The model under review builds one solid part; all positions refer to its coordinate system, in mm. A direction names the side the tool comes from. Give positions to 0.01 mm unless a question says otherwise; leave off trailing zeros. Order: outer loops, then holes, each group sorted by start corner. A loop starts at its lowest first (then second) coordinate and runs counter-clockwise, first axis right, second up.
```python
from build123d import *

# Parameters (mm, degrees)
F1_DEPTH    = 48
F2_DEPTH    = 10
F3_R        = 6.0205101074
F4_DEPTH    = 3
F5_T1_DEPTH = 30
F6_R        = 6


# Not quite as in the source:
# - a fillet or chamfer that OpenCascade refuses, or shapes differently, is made with other operations: its cross-section is extruded or revolved along the edge and cut away or added


with BuildPart() as f1:
    # F0 (on Top) → F1 (new body)
    with BuildSketch(Plane.XY):
        Polygon((20, 10), (0, 10), (-20, 10), (-20, 30), (-30, 30), (-30, 0), (0, 0), (30, 0), (30, 30), (20, 30), align=None)
    extrude(amount=F1_DEPTH)

    # F0 (on Top) → F2 (join)
    with BuildSketch(Plane.XY):
        Polygon((20, 10), (0, 10), (-20, 10), (-20, 30), (-30, 30), (-30, 0), (0, 0), (30, 0), (30, 30), (20, 30), align=None)
        Polygon((-30, 0), (-30, 30), (-45, 30), (-45, -18), (0, -18), (45, -18), (45, 30), (30, 30), (30, 0), (0, 0), align=None)
    extrude(amount=F2_DEPTH)

    # F3 (on Front) → F4 (join)
    with BuildSketch(Plane.XZ):
        with BuildLine():
            Line((14, 10), (14, 29))
            ThreePointArc((14, 29), (0, 43), (-14, 29))
            Line((-14, 29), (-14, 10))
            Line((-14, 10), (14, 10))
        make_face()
        with Locations((0, 29)):
            Circle(F3_R, mode=Mode.SUBTRACT)
    extrude(amount=F4_DEPTH)

    # F5: fillet of radius 25 on 2 edges, made by hand

    # F5_s2 → F5_t1 (join)
    with BuildSketch(Plane.XZ.offset(-30)):
        with BuildLine():
            ThreePointArc((30, 32.9128784748), (34.0834993366, 19.2198145372), (45, 10))
            Line((45, 10), (30, 10))
            Line((30, 10), (30, 32.9128784748))
        make_face()
        with BuildLine():
            ThreePointArc((-30, 32.9128784748), (-34.0834993366, 19.2198145372), (-45, 10))
            Line((-45, 10), (-30, 10))
            Line((-30, 10), (-30, 32.9128784748))
        make_face()
    extrude(amount=F5_T1_DEPTH)

    # F6
    f6_edges = [f1.edges().sort_by_distance(p)[0] for p in [
        (-45, -18, 5),
        (45, -18, 5),
    ]]
    fillet(f6_edges, radius=F6_R)


solid = f1.part
```
Item 1: Take a section at B-B (z = 3). Give the boundary of the cut face in (x, y), and give its area (3 significant figures).
Values found:
outline: (-45, -12) arc R6 ccw to (-39, -18) - (39, -18) arc R6 ccw to (45, -12) - (45, 30) - (20, 30) - (20, 10) - (-20, 10) - (-20, 30) - (-45, 30) - close
area: 3,500 mm2
Item 2: Draft analysis for pull direction Z (two halves, no side actions). For faces 5 (the flat face through (0, 9, 48)), 6 (the flat face through (30, 30, 19)), 7 (the flat face through (0, 0, 29)), state which applies: released by +Z, released by -Z, zero draft, split by the parting line, or undercut.
Values found:
face 5: released by +Z
face 6: zero draft
face 7: undercut
Item 3: For faces 1 (the flat face through (-20, 20, 24)), 2 (the flat face through (14, -1, 19)), 3 (the flat face through (-9, 0, 42)), 4 (the flat face through (-14, -1, 20)), list the 3-axis set-ups (+Z, -Z, +X, -X, +Y, -Y) from which the entire face can be reached by the end or side of a thin tool; tool diameter is ignored.
Values found:
face 1: +Z, -Z, +Y
face 2: +Z, +X, -Y
face 3: +Z, -Y
face 4: +Z, -X, -Y
Item 4: Take a section at C-C (y = 11). Give the boundary of the cut face in (x, z), and give its area (3 significant figures).
Values found:
outline: (-45, 0) - (-20, 0) - (-20, 48) - (-30, 48) - (-30, 32.91) arc R25 cw to (-45, 10) - close; (20, 0) - (45, 0) - (45, 10) arc R25 cw to (30, 32.91) - (30, 48) - (20, 48) - close
area: 1,450 mm2
Item 5: Clearance check with flat-ended pins moving along their axes: pin 1 Ø7 at (x, z) = (0, 29) entering from +Y; pin 2 Ø3.5 at (y, z) = (-1, 18.5) entering from +X; pin 3 Ø3.5 at (x, z) = (2, 26.5) entering from -Y. State where each tip first meets the part, or that it passes through.
Values found:
pin 1: stops at y = 10
pin 2: stops at x = 35.67
pin 3: stops at y = 0
Item 6: Take a section at D-D (x = 0). Give the boundary of the cut face in (y, z), and give its area (3 significant figures).
Values found:
outline: (-18, 0) - (10, 0) - (10, 48) - (0, 48) - (0, 43) - (-3, 43) - (-3, 35.02) - (0, 35.02) - (0, 22.98) - (-3, 22.98) - (-3, 10) - (-18, 10) - close
area: 723 mm2
Item 7: For line 1 (Z direction, x = 0, y = -1.1); line 2 (X direction, y = 25, z = 33); line 3 (Y direction, x = 10.5, z = 8), list the stretches that pass through material, from the lowest coordinate up.
Values found:
line 1: z = 0 to 22.98, 35.02 to 43
line 2: x = -30 to -20, 20 to 30
line 3: y = -18 to 10
Item 8: Take a section at A-A (y = -1). Give the boundary of the cut face in (x, z), and give its area (3 significant figures).
Values found:
outline: (-45, 0) - (45, 0) - (45, 10) - (14, 10) - (14, 29) arc R14 ccw to (-14, 29) - (-14, 10) - (-45, 10) - close; hole circle Ø12.04 at (0, 29)
area: 1,630 mm2
